from build123d import *

# Parameters (mm, degrees)
SKETCH2_W  = 16
SKETCH2_H  = 2.5
SLOT_DEPTH = 2.4


with BuildPart() as part:
    # BodySke → Base-Revolve (revolve)
    with BuildSketch(Plane.XY, mode=Mode.PRIVATE) as base_revolve_sk:
        Polygon((6, 5), (6, 8), (0, 8), (0, 0), (46, 0), (46, 5), align=None)
    revolve(base_revolve_sk.sketch.rotate(Axis((-25.4, 0, 0), (1, 0, 0)), 90), axis=Axis((-25.4, 0, 0), (1, 0, 0)))

    # Sketch2 → Slot (cut)
    with BuildSketch(Plane(origin=(0, 0, 0), x_dir=(0, 0, -1), z_dir=(1, 0, 0))):
        Rectangle(SKETCH2_W, SKETCH2_H)
    extrude(amount=SLOT_DEPTH, mode=Mode.SUBTRACT)


solid = part.part
The model under review builds one solid part; all positions refer to its coordinate system, in mm. A direction names the side the tool comes from. Round coordinates to 2 decimals unless told otherwise and drop trailing zeros. Loops run counter-clockwise (first coordinate to the right, second up) from the corner with the lowest first, then second, coordinate; pieces in that order, holes last. Notation, with made-up numbers: (61, 75) -> (74, 75) arc R17 cw to (74, 96) -> close; hole circle Ø1 at (1, 49.25). An arc over 180 degrees is marked (long way). Write item = value, one per line. Start each with the question number.
Item 1: Take a section at B-B on y = 0. Give the boundary of the cut face in (x, z), plus the area to 3 significant figures.
Item 2: Take a section at C-C on x = 21. Give the boundary of the cut face in (y, z).
Item 3: For faces 5 (the flat face through (1, -1.25, 0)), 6 (the flat face through (6, -0.1, -5.2)), 7 (the cylindrical face through (2.96, 3.06, 7.39)), list the 3-axis set-ups (+Z, -Z, +X, -X, +Y, -Y) from which the entire face can be reached by the end or side of a thin tool; tool diameter is ignored.
Item 4: To check wall thickness, follow L1, parallel to Y at x = 2, z = 6.25; L2, parallel to Y at x = 13.5, z = 0.25. State the ranges of each line that lie inside material, in increasing order.
Item 5: Take a section at A-A on z = 0. Give the boundary of the cut face in (x, y).
Item 6: Take a section at D-D on z = 6.5. Give the boundary of the cut face in (x, y).
Item 7: Mouldability with a two-part tool opening along Y and no side actions: class faces 1 (the flat face through (2.4, 0, 0)), 2 (the cylindrical face through (26, 0, -5)), 3 (the flat face through (46, 0, 0)), 4 (the flat face through (1, 1.25, 0)) as released by +Y, released by -Y, zero draft, split by the parting line, or undercut.
Item 8: Insertion check: pin 1 (1.2 mm diameter, centred on x = 1, z = -1, fed in from -Y); pin 2 (8 mm diameter, centred on x = 32, y = 0.5, fed in from -Z); pin 3 (4 mm diameter, centred on x = 7, y = -5.5, fed in from -Z); pin 4 (2.5 mm diameter, centred on x = 1.5, z = -0.5, fed in from +Y). Each pin has a flat end and moves straight along its axis. Give the tip position at first contact, or say it passes through.
Result:
q1.outline = (2.4, -8) -> (6, -8) -> (6, -5) -> (46, -5) -> (46, 5) -> (6, 5) -> (6, 8) -> (2.4, 8) -> close
q1.area = 458 mm²
q2.outline = circle Ø10 at (0, 0)
q3.face_5 = +Z, -Z, -X
q3.face_6 = +X
q3.face_7 = +X, -X
q4.L1 = -4.99 to -1.25, 1.25 to 4.99
q4.L2 = -4.99 to 4.99
q5.outline = (0, -8) -> (6, -8) -> (6, -5) -> (46, -5) -> (46, 5) -> (6, 5) -> (6, 8) -> (0, 8) -> (0, 1.25) -> (2.4, 1.25) -> (2.4, -1.25) -> (0, -1.25) -> close
q6.outline = (0, -4.66) -> (6, -4.66) -> (6, 4.66) -> (0, 4.66) -> (0, 1.25) -> (2.4, 1.25) -> (2.4, -1.25) -> (0, -1.25) -> close
q7.face_1 = undercut
q7.face_2 = split by the parting line
q7.face_3 = zero draft
q7.face_4 = undercut
q8.pin_1 = -7.99
q8.pin_2 = -5
q8.pin_3 = -7.06
q8.pin_4 = 8
